from build123d import *

# Parameters (mm, degrees)
SKETCH_1_R      = 5
SKETCH_1_R_2    = 2.5
EXTRUDE_1_DEPTH = 30
SKETCH_2_R      = 2
EXTRUDE_2_DEPTH = 6


with BuildPart() as part:
    # 草图1 → 凸台-拉伸1 (new body)
    with BuildSketch(Plane(origin=(0, 0, 0), x_dir=(1, 0, 0), z_dir=(0, 1, 0))):
        with Locations(Location((0, 0, 0), (0, 0, 270))):
            Circle(SKETCH_1_R)
        with Locations(Location((0, 0, 0), (0, 0, 270))):
            Circle(SKETCH_1_R_2, mode=Mode.SUBTRACT)
    extrude(amount=EXTRUDE_1_DEPTH)

    # 草图2 → 凸台-拉伸2 (add)
    with BuildSketch(Plane(origin=(0, 30, 0), x_dir=(1, 0, 0), z_dir=(0, 1, 0))):
        Polygon((0, 6.92820323), (-6, 3.464101615), (-6, -3.464101615), (0, -6.92820323), (6, -3.464101615), (6, 3.464101615), align=None)
        with Locations(Location((0, 0, 0), (0, 0, 270))):
            Circle(SKETCH_2_R, mode=Mode.SUBTRACT)
    extrude(amount=-EXTRUDE_2_DEPTH)


solid = part.part
Geometry: final body of the model. Coordinates: model frame, mm. A direction names the side the tool comes from. Round coordinates to 2 decimals unless told otherwise and drop trailing zeros. Order: outer loops, then holes, each group sorted by start corner. A loop starts at its lowest first (then second) coordinate and runs counter-clockwise, first axis right, second up. Notation, with made-up numbers: (70.25, 22.25) -> (106.25, 22.25) arc R34 cw to (106.25, 57.25) -> close; hole circle Ø10 at (61.25, 33). An arc over 180 degrees is marked (long way). Put each result on its own line as item: value. Start each with the question number.
Q1. Reachability of faces 5 (the flat face through (-0.9, 24, 5.1)), 6 (the flat face through (2.96, 27.04, 5.22)) from +Z, -Z, +X, -X, +Y, -Y: full face, straight path, thin tool, end or side. Return the list, or none.
Q2. First-contact query: pin 1 (6.5 mm diameter, centred on x = 0, z = 0, fed in from +Y); pin 2 (4.5 mm diameter, centred on x = 0, z = 0, fed in from -Y); pin 3 (2 mm diameter, centred on x = 3.5, y = 15, fed in from +Z); pin 4 (5 mm diameter, centred on x = 4.5, y = 6, fed in from -Z). Flat tips, straight axial feed; report the tip coordinate or a pass-through.
Q3. Section D-D on z = -4.5. Return the cut outline in (x, y).
Q4. Section A-A on z = 0. Return the cut outline in (x, y).
Q5. Section B-B on y = 25. Return the cut outline in (x, z), and give its area (3 significant figures).
Q6. Section C-C on x = -4.25. Return the cut outline in (y, z), and give its area (3 significant figures).
Q7. Line query: probe 1 along Z at (x, y) = (-1.5, 22.75); probe 2 along Z at (x, y) = (0, 7); probe 3 along X at (y, z) = (28.5, 0). Output: solid intervals per line, ascending.
Q8. Pull-direction query (X, two-part tool) for faces 1 (the flat face through (6, 27, 0)), 2 (the flat face through (-1, 24, -2)), 3 (the cylindrical face through (-2.44, 11.83, -0.54)), 4 (the flat face through (-1, 30, -2)); classes: +X half, -X half, draft (parallel to the pull), parting line (faces both ways), or undercut.
Ans:
1. face 5: -Y
1. face 6: +Z, +X, +Y, -Y
2. pin 1: stops at y = 30
2. pin 2: stops at y = 24
2. pin 3: stops at z = 4.33
2. pin 4: stops at z = -4.58
3. outline: (-4.21, 24) -> (-2.18, 24) -> (-2.18, 0) -> (2.18, 0) -> (2.18, 24) -> (4.21, 24) -> (4.21, 30) -> (-4.21, 30) -> close
4. outline: (-6, 24) -> (-5, 24) -> (-5, 0) -> (-2.5, 0) -> (-2.5, 24) -> (-2, 24) -> (-2, 30) -> (-6, 30) -> close; (2, 24) -> (2.5, 24) -> (2.5, 0) -> (5, 0) -> (5, 24) -> (6, 24) -> (6, 30) -> (2, 30) -> close
5. outline: (-6, -3.46) -> (0, -6.93) -> (6, -3.46) -> (6, 3.46) -> (0, 6.93) -> (-6, 3.46) -> close; hole circle Ø4 at (0, 0)
5. area: 112 mm2
6. outline: (0, -2.63) -> (24, -2.63) -> (24, -4.47) -> (30, -4.47) -> (30, 4.47) -> (24, 4.47) -> (24, 2.63) -> (0, 2.63) -> close
6. area: 180 mm2
7. probe 1: z = -4.77 to -2, 2 to 4.77
7. probe 2: z = -5 to -2.5, 2.5 to 5
7. probe 3: x = -6 to -2, 2 to 6
8. face 1: +X half
8. face 2: undercut
8. face 3: undercut
8. face 4: draft
